Autodesk Inventor part; units mm, degrees
ref_plane "YZ Plane" through (0, 0, 0) normal (1, 0, 0) x (0, 1, 0)
ref_plane "XZ Plane" through (0, 0, 0) normal (0, 1, 0) x (-1, 0, 0)
ref_plane "XY Plane" through (0, 0, 0) normal (0, 0, 1) x (1, 0, 0)
sketch "Sketch1" plane through (0, 0, 0) normal (0, 1, 0) x (-1, 0, 0)
  line L0 (0, 0) -> (19.05, 0)
  line L1 (19.05, 0) -> (19.05, -25.4)
  line L2 (19.05, -25.4) -> (0, -25.4)
  line L3 (0, -25.4) -> (0, 0)
  dimension "d0" = 19.05
  dimension "d1" = 25.4
extrude "Extrusion1" add sketch "Sketch1" along normal blind 25.4
sketch "Sketch2" plane through (-19.05, 0, 0) normal (0, 0, 1) x (1, 0, 0)
  circle A0 centre (9.525, 16.51) radius 6.35
  line L0 (0, 25.4) -> (19.05, 25.4)
  line L1 (3.175, 8.89) -> (15.875, 8.89)
  line L2 (15.875, 8.89) -> (15.875, 2.54)
  line L3 (15.875, 2.54) -> (3.175, 2.54)
  line L4 (3.175, 2.54) -> (3.175, 8.89)
  line L5 (0, 0) -> (0, 25.4)
  line L6 (19.05, 0) -> (19.05, 25.4)
  line L7 (19.05, 0) -> (0, 0)
  dimension "d4" = 12.7
  dimension "d5" = 8.89
  dimension "d6" = 12.7
  dimension "d7" = 19.05
  dimension "d8" = 6.35
  dimension "d9" = 3.175
  dimension "d10" = 3.175
  dimension "d16" = 2.54
extrude "Extrusion2" cut sketch "Sketch2" against normal blind 25.4 contours A0 | L1 L2 L3 L4
sketch "Sketch3" plane through (0, 0, 0) normal (0, -1, 0) x (1, 0, 0)
  circle A0 centre (-9.525, -12.7) radius 6.35
  point P0 (0, 0)
  dimension "d13" = 12.7
extrude "Extrusion3" cut sketch "Sketch3" against normal blind 3.175
properties part number "Pivot Poin 3"
Read the model definition and answer for the solid it produces. Units are mm, in the model's axes. A direction names the side the tool comes from. Coordinates: 2 decimals unless noted, no trailing zeros. Order: outer loops, then holes, each group sorted by start corner. A loop starts at its lowest first (then second) coordinate and runs counter-clockwise, first axis right, second up. Notation, with made-up numbers: M 1,62.5 L 10,62.5 A28 cw 10,101.5 Z; hole C 9.25,-18.5 d3. An arc over 180 degrees is marked long. Put each result on its own line as item: value. Start each with the question number.
Item 1: Section C-C, the plane x = -7 is taken. Determine the outline of the cut face in (y, z), plus the area to 3 significant figures.
Item 2: Section B-B, the plane z = -22.25 is taken. Determine the outline of the cut face in (x, y) (3 decimals), plus the area to 3 significant figures.
Item 3: Consider probe 1 along Y at (x, z) = (-9.5, -19.75); probe 2 along X at (y, z) = (4.75, -8.75) (3 decimals); probe 3 along Y at (x, z) = (-4, -19.75). Determine where each line is inside the solid, lowest interval first. Write a range as [from, to].
Item 4: Section A-A, the plane y = 16.51 is taken. Determine the outline of the cut face in (x, z) (3 decimals), plus the area to 3 significant figures.
Item 5: Given pin 1 Ø10 at (x, z) = (-9.525, -12.7) entering from -Y, flat-ended and moving along its own axis, determine where the tip first touches the part or whether it passes through.
Item 6: Section D-D, the plane z = -9.75 is taken. Determine the outline of the cut face in (x, y) (3 decimals).
Item 7: The mould has two halves that part along Y. Classify faces 1 (the face through (-9, 25.4, -13)), 2 (the face through (-9, 10, 0)), 3 (the face through (-9, 2.54, -3)): +Y half, -Y half, draft (parallel to the pull), parting line (faces both ways), or undercut.
Item 8: For faces 4 (the face through (0, 13, -13)), 5 (the face through (-3.66, 1.25, -15.13)), 6 (the face through (-9, 2.54, -22)), determine the directions among +Z, -Z, +X, -X, +Y, -Y from which every point of the face is accessible in a straight line to the end or side of a thin tool.
Computed:
1. outline: M 0,-25.4 L 2.54,-25.4 L 2.54,-18.53 L 0,-18.53 Z; M 0,-6.87 L 2.54,-6.87 L 2.54,0 L 0,0 Z; M 8.89,-25.4 L 10.68,-25.4 L 10.68,0 L 8.89,0 Z; M 22.34,-25.4 L 25.4,-25.4 L 25.4,0 L 22.34,0 Z
1. area: 158 mm2
2. outline: M -19.05,0 L 0,0 L 0,25.4 L -19.05,25.4 Z; hole M -15.875,2.54 L -3.175,2.54 L -3.175,8.89 L -15.875,8.89 Z; hole C -9.525,16.51 d12.7
2. area: 277 mm2
3. probe 1: y = [0, 2.54], [8.89, 10.16], [22.86, 25.4]
3. probe 2: x = [-19.05, -15.875], [-3.175, 0]
3. probe 3: y = [0, 2.54], [8.89, 13.38], [19.64, 25.4]
4. outline: M -19.05,-25.4 L -15.875,-25.4 L -15.875,0 L -19.05,0 Z; M -3.175,-25.4 L 0,-25.4 L 0,0 L -3.175,0 Z
4. area: 161 mm2
5. pin 1: stops at y = 8.89
6. outline: M -19.05,0 L -15.148,0 L -15.148,2.54 L -15.875,2.54 L -15.875,8.89 L -3.175,8.89 L -3.175,2.54 L -3.902,2.54 L -3.902,0 L 0,0 L 0,25.4 L -19.05,25.4 Z; hole C -9.525,16.51 d12.7
7. face 1: +Y half
7. face 2: draft
7. face 3: undercut
8. face 4: +Z, -Z, +X, +Y, -Y
8. face 5: -Y
8. face 6: +Z, -Z
